from build123d import *

# Parameters (mm, degrees)
F1_DEPTH = 1016
F2_W     = 685.8
F2_H     = 367.284
F3_DEPTH = 19.051
F4_R     = 47.625
F5_DEPTH = 19.051


with BuildPart() as f1:
    # F0 (on Front) → F1 (new body)
    with BuildSketch(Plane.XZ):
        Polygon((-19.05, 7.890768), (0, 0), (0, 406.4), (-19.05, 406.4), align=None)
    extrude(amount=F1_DEPTH)

    # F2 (on face) → F3 (cut, through all)
    with BuildSketch(Plane(origin=(-19.05, 0, 0), x_dir=(0, -1, 0), z_dir=(-1, 0, 0))):
        with Locations((508, 207.145384)):
            Rectangle(F2_W, F2_H)
    extrude(amount=-F3_DEPTH, mode=Mode.SUBTRACT)

    # F4 (on face) → F5 (cut, through all)
    with BuildSketch(Plane(origin=(-19.05, 0, 0), x_dir=(0, -1, 0), z_dir=(-1, 0, 0))):
        with Locations((82.55, 306.772692)):
            Circle(F4_R)
        with Locations((82.55, 107.518076)):
            Circle(F4_R)
        with Locations((933.45, 306.772692)):
            Circle(F4_R)
        with Locations((933.45, 107.518076)):
            Circle(F4_R)
    extrude(amount=-F5_DEPTH, mode=Mode.SUBTRACT)


solid = f1.part
The model under review builds one solid part; all positions refer to its coordinate system, in mm. A direction names the side the tool comes from. Coordinates: 2 decimals unless noted, no trailing zeros. Write each loop counter-clockwise with the first axis right and the second up, starting at its lowest first coordinate (ties: lowest second). Pieces come first, ordered by that corner, then holes. Notation, with made-up numbers: (17, 68) - (51, 68) arc R29 cw to (51, 100) - close; hole circle Ø2 at (74, -34). An arc over 180 degrees is marked (long way). Answer as a JSON object with one key per item and string values. Group by question number.
1. Mouldability with a two-part tool opening along Y and no side actions: class faces 3 (the face through (-9.658, -126.543, 288.532)), 4 (the face through (-10, -1016, 206)), 5 (the face through (-9, -501, 406.4)), 6 (the face through (-10, -165.1, 205)) as pulls with the +Y half, pulls with the -Y half, needs draft (parallel to the pull), parting line crosses it, or undercut.
2. Add section A-A (z = 202). Give the boundary of the cut face in (x, y), plus the area to 3 significant figures.
3. Add section D-D (x = -4.25). Give the boundary of the cut face in (y, z) (3 decimals).
4. To check wall thickness, follow probe 1 along Y at (x, z) = (-1, 166.5); probe 2 along Y at (x, z) = (-1.25, 286.5); probe 3 along Z at (x, y) = (-6.25, -933.45). State the ranges of each line that lie inside material, in increasing order.
5. Machinability: for faces 1 (the face through (-10, -503, 390.787)), 2 (the face through (0, -506, 22)), which of the approach directions +Z, -Z, +X, -X, +Y, -Y give a long, thin tool a straight path to every point of the face, cutting with its end or side? Answer none if there is none.
6. Clearance check with flat-ended pins moving along their axes: pin 1 Ø1.5 at (x, z) = (-8.5, 161.5) entering from +Y; pin 2 Ø3 at (x, y) = (-12.5, -571.5) entering from -Z; pin 3 Ø9.5 at (x, y) = (-12.5, -600) entering from -Z. State where each tip first meets the part, or that it passes through.
7. Add section C-C (y = -933.45). Give the boundary of the cut face in (x, z), plus the area to 3 significant figures.
8. Add section B-B (y = -267). Give the boundary of the cut face in (x, z), plus the area to 3 significant figures.
Findings:
{
 "1": {"face 3": "undercut", "face 4": "pulls with the -Y half", "face 5": "needs draft", "face 6": "undercut"},
 "2": {"outline": "(-19.05, -1016) - (0, -1016) - (0, -850.9) - (-19.05, -850.9) - close; (-19.05, -165.1) - (0, -165.1) - (0, 0) - (-19.05, 0) - close", "area": "6,290 mm²"},
 "3": {"outline": "(-1016, 1.76) - (0, 1.76) - (0, 406.4) - (-1016, 406.4) - close; hole circle Ø95.25 at (-933.45, 107.518); hole circle Ø95.25 at (-933.45, 306.773); hole (-850.9, 23.503) - (-165.1, 23.503) - (-165.1, 390.787) - (-850.9, 390.787) - close; hole circle Ø95.25 at (-82.55, 107.518); hole circle Ø95.25 at (-82.55, 306.773)"},
 "4": {"probe 1": "-1016 to -850.9, -165.1 to 0", "probe 2": "-1016 to -976.54, -890.36 to -850.9, -165.1 to -125.64, -39.46 to 0", "probe 3": "2.59 to 59.89, 155.14 to 259.15, 354.4 to 406.4"},
 "5": {"face 1": "+X, -X", "face 2": "+Z, -Z, +X, +Y, -Y"},
 "6": {"pin 1": "y = 0", "pin 2": "z = 4.56", "pin 3": "z = 3.21"},
 "7": {"outline": "(-19.05, 7.89) - (0, 0) - (0, 59.89) - (-19.05, 59.89) - close; (-19.05, 155.14) - (0, 155.14) - (0, 259.15) - (-19.05, 259.15) - close; (-19.05, 354.4) - (0, 354.4) - (0, 406.4) - (-19.05, 406.4) - close", "area": "4,040 mm²"},
 "8": {"outline": "(-19.05, 7.89) - (0, 0) - (0, 23.5) - (-19.05, 23.5) - close; (-19.05, 390.79) - (0, 390.79) - (0, 406.4) - (-19.05, 406.4) - close", "area": "670 mm²"}
}
